```python
from build123d import *

# Parameters (mm, degrees)
EXTRUDE_1_DEPTH     = 10
SKETCH_3_R          = 2
CUT_EXTRUDE_2_DEPTH = 4
SKETCH_4_R          = 2.25
CUT_EXTRUDE_3_DEPTH = 3.2


with BuildPart() as part:
    # 草图1 → 凸台-拉伸1 (new body)
    with BuildSketch(Plane.XY):
        with BuildLine():
            Line((0, 23), (3, 23))
            Line((3, 23), (3, 10))
            Line((3, 10), (0, 10))
            ThreePointArc((0, 10), (-10, 0), (0, -10))
            Line((0, -10), (3, -10))
            Line((3, -10), (3, -23))
            Line((3, -23), (0, -23))
            Line((0, -23), (0, -13))
            ThreePointArc((0, -13), (-13, 0), (0, 13))
            Line((0, 13), (0, 23))
        make_face()
    extrude(amount=EXTRUDE_1_DEPTH)

    # 草图3 → 切除-拉伸2 (cut, through all)
    with BuildSketch(Plane.ZY):
        with Locations((5, 18)):
            Circle(SKETCH_3_R)
    extrude(amount=-CUT_EXTRUDE_2_DEPTH, mode=Mode.SUBTRACT)

    # 草图4 → 切除-拉伸3 (cut)
    with BuildSketch(Plane.ZY):
        with Locations((5, -18)):
            Circle(SKETCH_4_R)
    extrude(amount=-CUT_EXTRUDE_3_DEPTH, mode=Mode.SUBTRACT)


solid = part.part
```
For this review, take the finished solid that the model builds, in its own axes (mm). A direction names the side the tool comes from. Coordinates: 2 decimals unless noted, no trailing zeros. Loops run counter-clockwise (first coordinate to the right, second up) from the corner with the lowest first, then second, coordinate; pieces in that order, holes last. Notation, with made-up numbers: (23.5, 22.25) -> (53.5, 22.25) arc R31 cw to (53.5, 47.25) -> close; hole circle Ø2 at (66.25, 18). An arc over 180 degrees is marked (long way). Return JSON: item names as keys, results as strings. Group by question number.
(1) Consider section A-A, the plane y = -18. Give the boundary of the cut face in (x, z).
(2) Consider section B-B, the plane x = 0.5. Give the boundary of the cut face in (y, z), plus the area to 3 significant figures.
(3) Consider section C-C, the plane z = 5. Give the boundary of the cut face in (x, y), plus the area to 3 significant figures.
(4) Consider section D-D, the plane z = 7.75. Give the boundary of the cut face in (x, y), plus the area to 3 significant figures.
(5) For pin 1 Ø3 at (x, z) = (-4, 4) entering from +Y; pin 2 Ø3 at (y, z) = (-20, 4) entering from -X; pin 3 Ø4 at (y, z) = (-18, 5) entering from -X; pin 4 Ø3 at (y, z) = (-9.5, 4.5) entering from -X, all flat-tipped, find the tip position at first contact; note any pin that passes through.
(6) Tool access review of faces 5 (the flat face through (0, 15.7, 4.9)), 6 (the flat face through (0, -20.3, 3.8)), 7 (the flat face through (1, -10, 5)): name each direction out of +Z, -Z, +X, -X, +Y, -Y from which nothing blocks a thin tool from reaching the whole face with its end or side.
(7) To check wall thickness, follow L1, parallel to Y at x = 0.9, z = 5; L2, parallel to Y at x = -0.25, z = 3.5; L3, parallel to Y at x = 1.75, z = 2. State the ranges of each line that lie inside material, in increasing order.
(8) Mouldability with a two-part tool opening along Y and no side actions: class faces 1 (the flat face through (3, 15, 5)), 2 (the flat face through (2, 10, 5)), 3 (the flat face through (1, 23, 5)), 4 (the cylindrical face through (1, 20, 5)) as pulls with the +Y half, pulls with the -Y half, needs draft (parallel to the pull), parting line crosses it, or undercut.
Results below:
{
 "1": {"outline": "(0, 0) -> (3, 0) -> (3, 2.75) -> (0, 2.75) -> close; (0, 7.25) -> (3, 7.25) -> (3, 10) -> (0, 10) -> close"},
 "2": {"outline": "(-23, 0) -> (-10, 0) -> (-10, 10) -> (-23, 10) -> close; (10, 0) -> (23, 0) -> (23, 10) -> (10, 10) -> close; hole circle Ø4.5 at (-18, 5); hole circle Ø4 at (18, 5)", "area": "232 mm2"},
 "3": {"outline": "(0, -23) -> (3, -23) -> (3, -20.25) -> (0, -20.25) -> close; (0, -15.75) -> (3, -15.75) -> (3, -10) -> (0, -10) arc R10 cw to (0, 10) -> (3, 10) -> (3, 16) -> (0, 16) -> (0, 13) arc R13 ccw to (0, -13) -> close; (0, 20) -> (3, 20) -> (3, 23) -> (0, 23) -> close", "area": "161 mm2"},
 "4": {"outline": "(0, -23) -> (3, -23) -> (3, -10) -> (0, -10) arc R10 cw to (0, 10) -> (3, 10) -> (3, 23) -> (0, 23) -> (0, 13) arc R13 ccw to (0, -13) -> close", "area": "186 mm2"},
 "5": {"pin 1": "stops at y = 12.76", "pin 2": "stops at x = 0", "pin 3": "passes through", "pin 4": "stops at x = -10.25"},
 "6": {"face 5": "+Z, -Z, -X, +Y", "face 6": "+Z, -Z, -X, -Y", "face 7": "+Z, -Z, +X"},
 "7": {"L1": "y = -23 to -20.25, -15.75 to -10, 10 to 16, 20 to 23", "L2": "y = -13 to -10, 10 to 13", "L3": "y = -23 to -10, 10 to 23"},
 "8": {"face 1": "needs draft", "face 2": "undercut", "face 3": "pulls with the +Y half", "face 4": "undercut"}
}
